The model under review builds one solid part; all positions refer to its coordinate system, in mm. A direction names the side the tool comes from. Coordinates: 2 decimals unless noted, no trailing zeros. Order: outer loops, then holes, each group sorted by start corner. A loop starts at its lowest first (then second) coordinate and runs counter-clockwise, first axis right, second up. Notation, with made-up numbers: (-25, -13) -> (25, -13) arc R5 cw to (25, -7) -> close; hole circle Ø2 at (47, -28). An arc over 180 degrees is marked (long way). Use one line per item in the form item = value.
from build123d import *

# Parameters (mm, degrees)
F1_DEPTH = 30
F2_R     = 5
F3_W     = 124.640293
F3_H     = 81.299469
F4_DEPTH = 17.5
F5_R     = 1.5
F6_DEPTH = 22.5


with BuildPart() as f1:
    # F0 (on Right) → F1 (new body, symmetric)
    with BuildSketch(Plane.YZ):
        with BuildLine():
            Line((-100, -47.343845), (100, -47.343845))
            Line((100, -47.343845), (100, 52.656155))
            Line((100, 52.656155), (-46.951734, -17.113248))
            ThreePointArc((-46.951734, -17.113248), (-69.557005, -13.302077), (-73.732945, 9.238661))
            Line((-73.732945, 9.238661), (-53.972553, 52.656155))
            Line((-53.972553, 52.656155), (-92.148267, 52.656155))
            Line((-92.148267, 52.656155), (-100, -47.343845))
        make_face()
    extrude(amount=F1_DEPTH, both=True)

    # F2
    f2_edges = [f1.edges().sort_by_distance(p)[0] for p in [
        (0, -92.148267, 52.656155),
        (0, 100, 52.656155),
        (30, 26.524133, 17.771454),
        (-30, 26.524133, 17.771454),
        (30, 100, 2.656155),
        (-30, 100, 2.656155),
        (30, -96.074133, 2.656155),
        (-30, -96.074133, 2.656155),
    ]]
    fillet(f2_edges, radius=F2_R)

    # F3 (on Right) → F4 (cut, symmetric)
    with BuildSketch(Plane.YZ):
        with Locations((27.194251, 0.991457)):
            Rectangle(F3_W, F3_H)
    extrude(amount=F4_DEPTH, both=True, mode=Mode.SUBTRACT)

    # F5 (on Right) → F6 (cut, symmetric)
    with BuildSketch(Plane.YZ):
        with Locations((37.958637, 12.46403)):
            Circle(F5_R)
    extrude(amount=F6_DEPTH, both=True, mode=Mode.SUBTRACT)


solid = f1.part
Item 1: We need section A-A (x = -9.5). Write out the cut boundary in (y, z).
Results found:
outline = (-100, -47.34) -> (100, -47.34) -> (100, 44.75) arc R5 ccw to (92.86, 49.26) -> (76.8, 41.64) -> (89.51, 41.64) -> (89.51, -39.66) -> (-35.13, -39.66) -> (-35.13, -11.5) -> (-46.95, -17.11) arc R20 cw to (-73.73, 9.24) -> (-53.97, 52.66) -> (-87.53, 52.66) arc R5 ccw to (-92.51, 48.05) -> close
Item 2: Clearance check with flat-ended pins moving along their axes: pin 1 (3 mm diameter, centred on x = 10, z = 15, fed in from -Y); pin 2 (12 mm diameter, centred on x = 9.5, z = -26.5, fed in from -Y); pin 3 (10.5 mm diameter, centred on x = -2, z = -9.5, fed in from -Y). State where each tip first meets the part, or that it passes through.
Results found:
pin_1 = -95.22
pin_2 = -98.83
pin_3 = -97.44
Item 3: Tool access review of faces 1 (the face through (-28.496, 22.585, 14.323)), 2 (the face through (28.496, 22.585, 14.323)), 3 (the face through (28.496, -65.012, 31.842)), 4 (the face through (0, 89.514, 0)): name each direction out of +Z, -Z, +X, -X, +Y, -Y from which nothing blocks a thin tool from reaching the whole face with its end or side.
Results found:
face_1 = +Z, -X
face_2 = +Z, +X
face_3 = +X
face_4 = none
Item 4: Draft analysis for pull direction Y (two halves, no side actions). For faces 5 (the face through (-0.42, -90.96, 51.29)), 6 (the face through (0, 26, -39.658)), 7 (the face through (-30, -1, -8)), state which applies: released by +Y, released by -Y, zero draft, split by the parting line, or undercut.
Results found:
face_5 = released by -Y
face_6 = undercut
face_7 = zero draft
Item 5: To check wall thickness, follow L1, parallel to X at y = 69, z = -25; L2, parallel to Z at x = 16.5, y = 62; L3, parallel to Y at x = 5.5, z = 6. State the ranges of each line that lie inside material, in increasing order. Write a range as from..to.
Results found:
L1 = -30..-17.5, 17.5..30
L2 = -47.34..-39.66
L3 = -95.81..-74.88, 89.51..100
